For this review, take the finished solid that the model builds, in its own axes (mm). A direction names the side the tool comes from. Coordinates: 2 decimals unless noted, no trailing zeros. Loops run counter-clockwise (first coordinate to the right, second up) from the corner with the lowest first, then second, coordinate; pieces in that order, holes last. Notation, with made-up numbers: (-19.75, 4.25) -> (14.25, 4.25) arc R18 cw to (14.25, 16.25) -> close; hole circle Ø9 at (9, 67.25). An arc over 180 degrees is marked (long way). One line per item, written item: value.
from build123d import *

# Parameters (mm, degrees)
F1_DEPTH = 101.6
F2_W     = 3.175
F2_H     = 12.7
F3_DEPTH = 12.7
F5_D     = 6.35
F6_R     = 5.08


with BuildPart() as f1:
    # F0 (on Front) → F1 (new body)
    with BuildSketch(Plane.XZ):
        with BuildLine():
            Line((17.4625, 15.875), (-17.4625, 15.875))
            ThreePointArc((-17.4625, 15.875), (-24.197692, 13.085192), (-26.9875, 6.35))
            Line((-26.9875, 6.35), (-26.9875, -6.35))
            ThreePointArc((-26.9875, -6.35), (-24.197692, -13.085192), (-17.4625, -15.875))
            Line((-17.4625, -15.875), (17.4625, -15.875))
            ThreePointArc((17.4625, -15.875), (24.197692, -13.085192), (26.9875, -6.35))
            Line((26.9875, -6.35), (26.9875, 6.35))
            ThreePointArc((26.9875, 6.35), (24.197692, 13.085192), (17.4625, 15.875))
        make_face()
        with BuildLine():
            ThreePointArc((-23.8125, 6.35), (-21.952628, 10.840128), (-17.4625, 12.7))
            Line((-17.4625, 12.7), (17.4625, 12.7))
            ThreePointArc((17.4625, 12.7), (21.952628, 10.840128), (23.8125, 6.35))
            Line((23.8125, 6.35), (23.8125, -6.35))
            ThreePointArc((23.8125, -6.35), (21.952628, -10.840128), (17.4625, -12.7))
            Line((17.4625, -12.7), (-17.4625, -12.7))
            ThreePointArc((-17.4625, -12.7), (-21.952628, -10.840128), (-23.8125, -6.35))
            Line((-23.8125, -6.35), (-23.8125, 6.35))
        make_face(mode=Mode.SUBTRACT)
    extrude(amount=F1_DEPTH)

    # F2 (on face) → F3 (join)
    with BuildSketch(Plane.XY.offset(15.875)):
        with Locations((-3.175, -50.8)):
            Rectangle(F2_W, F2_H)
        with Locations((3.175, -50.8)):
            Rectangle(F2_W, F2_H)
    extrude(amount=F3_DEPTH)

    # F5 (through all)
    with Locations(Plane.YZ.offset(4.7625)):
        with Locations((-50.8, 22.225)):
            Hole(F5_D / 2)

    # F6
    f6_edges = [f1.edges().sort_by_distance(p)[0] for p in [
        (-3.175, -57.15, 28.575),
        (3.175, -57.15, 28.575),
        (3.175, -44.45, 28.575),
        (-3.175, -44.45, 28.575),
    ]]
    fillet(f6_edges, radius=F6_R)


solid = f1.part
1. Insertion check: pin 1 Ø2.5 at (x, z) = (-4, 18) entering from -Y; pin 2 Ø2.5 at (x, z) = (2.5, 19) entering from +Y; pin 3 Ø6.5 at (y, z) = (-53.5, 22.5) entering from +X; pin 4 Ø5.5 at (y, z) = (-50.8, 22.225) entering from -X. Each pin has a flat end and moves straight along its axis. Give the tip position at first contact, or say it passes through.
Return value:
pin 1: stops at y = -57.15
pin 2: stops at y = -44.45
pin 3: stops at x = 4.76
pin 4: passes through
2. To check wall thickness, follow probe 1 along Z at (x, y) = (-4.05, -50.8) (3 decimals); probe 2 along Z at (x, y) = (-7, -94) (3 decimals); probe 3 along Z at (x, y) = (2, -50) (3 decimals). State the ranges of each line that lie inside material, in increasing order. Write a range as from..to.
Return value:
probe 1: z = -15.875..-12.7, 12.7..19.05, 25.4..28.575
probe 2: z = -15.875..-12.7, 12.7..15.875
probe 3: z = -15.875..-12.7, 12.7..19.152, 25.298..28.575
3. Take a section at B-B, the plane z = 18. Give the boundary of the cut face in (x, y), and give its area (3 significant figures).
Return value:
outline: (-4.76, -57.15) -> (-1.59, -57.15) -> (-1.59, -44.45) -> (-4.76, -44.45) -> close; (1.59, -57.15) -> (4.76, -57.15) -> (4.76, -44.45) -> (1.59, -44.45) -> close
area: 80.6 mm2
4. Take a section at D-D, the plane x = -19. Give the boundary of the cut face in (y, z).
Return value:
outline: (-101.6, -15.75) -> (0, -15.75) -> (0, -12.51) -> (-101.6, -12.51) -> close; (-101.6, 12.51) -> (0, 12.51) -> (0, 15.75) -> (-101.6, 15.75) -> close
5. The part is to be moulded in two halves that separate along Y. For faces 1 (the flat face through (-3, -57.15, 20)), 2 (the cylindrical face through (-3.2, -53.83, 23.18)), 3 (the cylindrical face through (-24.27, -50.09, -13.01)), say which applies: pulls with the +Y half, pulls with the -Y half, needs draft (parallel to the pull), parting line crosses it, or undercut.
Return value:
face 1: pulls with the -Y half
face 2: undercut
face 3: needs draft
6. For faces 4 (the flat face through (3, -44.45, 20)), 5 (the flat face through (-23.812, -50, 0)), 6 (the flat face through (-4.762, -52, 19)), list the 3-axis set-ups (+Z, -Z, +X, -X, +Y, -Y) from which the entire face can be reached by the end or side of a thin tool; tool diameter is ignored.
Return value:
face 4: +Z, +X, -X, +Y
face 5: +Y, -Y
face 6: +Z, -X, +Y, -Y
7. Take a section at A-A, the plane y = -50.8. Give the number of separate pieces and of enclosed holes in the cut face, and give its area (3 significant figures).
Return value:
separate pieces: 3
enclosed holes: 1
area: 501 mm2
